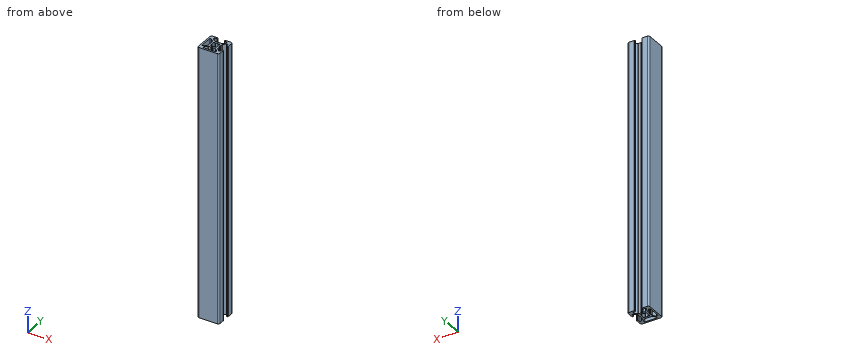
```python
from build123d import *

# Parameters (mm, degrees)
EXTRUDE1_DEPTH = 250


with BuildPart() as part:
    # Sketch1 → Extrude1 (new body)
    with BuildSketch(Plane.XY):
        with BuildLine():
            Line((-8.5, -10), (8.5, -10))
            ThreePointArc((8.5, -10), (9.560660172, -9.560660172), (10, -8.5))
            Line((10, -8.5), (10, -3.7))
            ThreePointArc((10, -3.7), (9.941421356, -3.558578644), (9.8, -3.5))
            Line((9.8, -3.5), (9.7, -3.5))
            ThreePointArc((9.7, -3.5), (9.558578644, -3.441421356), (9.5, -3.3))
            Line((9.5, -3.3), (9.5, -3.2))
            ThreePointArc((9.5, -3.2), (9.441421356, -3.058578644), (9.3, -3))
            Line((9.3, -3), (9, -3))
            ThreePointArc((9, -3), (8.646446609, -3.146446609), (8.5, -3.5))
            Line((8.5, -3.5), (8.5, -5.500000208))
            ThreePointArc((8.5, -5.500000208), (8.353553391, -5.853553598), (8, -6.000000208))
            Line((8, -6.000000208), (7.267767022, -6.000000208))
            ThreePointArc((7.267767022, -6.000000208), (7.076425294, -5.961939969), (6.914213614, -5.853553581))
            Line((6.914213614, -5.853553581), (4.646446828, -3.585786575))
            ThreePointArc((4.646446828, -3.585786575), (4.538060465, -3.423574906), (4.500000236, -3.232233201))
            Line((4.500000236, -3.232233201), (4.500000236, -0.953589838))
            ThreePointArc((4.500000236, -0.953589838), (4.493185401, -0.901826029), (4.473205317, -0.853589838))
            Line((4.473205317, -0.853589838), (4.038120021, -0.1))
            ThreePointArc((4.038120021, -0.1), (4.011325101, 0), (4.038120021, 0.1))
            Line((4.038120021, 0.1), (4.473205317, 0.853589838))
            ThreePointArc((4.473205317, 0.853589838), (4.493185401, 0.901826029), (4.500000236, 0.953589838))
            Line((4.500000236, 0.953589838), (4.500000236, 3.232233262))
            ThreePointArc((4.500000236, 3.232233262), (4.538060467, 3.423574973), (4.646446837, 3.585786644))
            Line((4.646446837, 3.585786644), (6.914213678, 5.853553596))
            ThreePointArc((6.914213678, 5.853553596), (7.076425355, 5.961939978), (7.267767077, 6.000000214))
            Line((7.267767077, 6.000000214), (8.000000112, 6.000000214))
            ThreePointArc((8.000000112, 6.000000214), (8.353553502, 5.853553604), (8.500000112, 5.500000214))
            Line((8.500000112, 5.500000214), (8.500000112, 3.5))
            ThreePointArc((8.500000112, 3.5), (8.646446721, 3.146446609), (9.000000112, 3))
            Line((9.000000112, 3), (9.300000112, 3))
            ThreePointArc((9.300000112, 3), (9.441421468, 3.058578644), (9.500000112, 3.2))
            Line((9.500000112, 3.2), (9.500000112, 3.3))
            ThreePointArc((9.500000112, 3.3), (9.558578756, 3.441421356), (9.700000112, 3.5))
            Line((9.700000112, 3.5), (9.8, 3.5))
            ThreePointArc((9.8, 3.5), (9.941421356, 3.558578644), (10, 3.7))
            Line((10, 3.7), (10, 8.5))
            ThreePointArc((10, 8.5), (9.560660172, 9.560660172), (8.5, 10))
            Line((8.5, 10), (3.7, 10))
            ThreePointArc((3.7, 10), (3.558578644, 9.941421356), (3.5, 9.8))
            Line((3.5, 9.8), (3.5, 9.7))
            ThreePointArc((3.5, 9.7), (3.441421356, 9.558578644), (3.3, 9.5))
            Line((3.3, 9.5), (3.2, 9.5))
            ThreePointArc((3.2, 9.5), (3.058578644, 9.441421356), (3, 9.3))
            Line((3, 9.3), (3, 9.000000069))
            ThreePointArc((3, 9.000000069), (3.146446609, 8.646446678), (3.5, 8.500000069))
            Line((3.5, 8.500000069), (5.550000287, 8.500000069))
            ThreePointArc((5.550000287, 8.500000069), (5.903553677, 8.353553459), (6.050000287, 8.000000069))
            Line((6.050000287, 8.000000069), (6.050000287, 7.267766898))
            ThreePointArc((6.050000287, 7.267766898), (6.011940051, 7.076425176), (5.903553669, 6.914213499))
            Line((5.903553669, 6.914213499), (3.635786717, 4.646446658))
            ThreePointArc((3.635786717, 4.646446658), (3.473575046, 4.538060288), (3.282233335, 4.500000057))
            Line((3.282233335, 4.500000057), (1.003589985, 4.500000057))
            ThreePointArc((1.003589985, 4.500000057), (0.951826176, 4.493185222), (0.903589985, 4.473205138))
            Line((0.903589985, 4.473205138), (0.150000146, 4.038119841))
            ThreePointArc((0.150000146, 4.038119841), (0.050000146, 4.011324922), (-0.049999854, 4.038119841))
            Line((-0.049999854, 4.038119841), (-0.803589692, 4.473205138))
            ThreePointArc((-0.803589692, 4.473205138), (-0.851825883, 4.493185222), (-0.903589692, 4.500000057))
            Line((-0.903589692, 4.500000057), (-3.182233104, 4.500000057))
            ThreePointArc((-3.182233104, 4.500000057), (-3.37357482, 4.538060291), (-3.535786494, 4.646446666))
            Line((-3.535786494, 4.646446666), (-5.803553391, 6.914213562))
            ThreePointArc((-5.803553391, 6.914213562), (-5.911939766, 7.076425237), (-5.95, 7.267766953))
            Line((-5.95, 7.267766953), (-5.95, 8))
            ThreePointArc((-5.95, 8), (-5.803553391, 8.353553391), (-5.45, 8.5))
            Line((-5.45, 8.5), (-3.5, 8.5))
            ThreePointArc((-3.5, 8.5), (-3.146446609, 8.646446609), (-3, 9))
            Line((-3, 9), (-3, 9.3))
            ThreePointArc((-3, 9.3), (-3.058578644, 9.441421356), (-3.2, 9.5))
            Line((-3.2, 9.5), (-3.35, 9.5))
            ThreePointArc((-3.35, 9.5), (-3.491421356, 9.558578644), (-3.55, 9.7))
            Line((-3.55, 9.7), (-3.55, 9.8))
            ThreePointArc((-3.55, 9.8), (-3.608578644, 9.941421356), (-3.75, 10))
            Line((-3.75, 10), (-8.5, 10))
            ThreePointArc((-8.5, 10), (-9.560660172, 9.560660172), (-10, 8.5))
            Line((-10, 8.5), (-10, -8.5))
            ThreePointArc((-10, -8.5), (-9.560660172, -9.560660172), (-8.5, -10))
        make_face()
        with BuildLine():
            Line((-5.500000147, -8.500000123), (5.500000242, -8.500000123))
            ThreePointArc((5.500000242, -8.500000123), (5.853553633, -8.353553514), (6.000000242, -8.000000123))
            Line((6.000000242, -8.000000123), (6.000000242, -7.267766878))
            ThreePointArc((6.000000242, -7.267766878), (5.961940006, -7.076425156), (5.853553624, -6.914213479))
            Line((5.853553624, -6.914213479), (3.585786637, -4.646446602))
            ThreePointArc((3.585786637, -4.646446602), (3.423574966, -4.538060233), (3.232233255, -4.500000001))
            Line((3.232233255, -4.500000001), (0.953589836, -4.500000001))
            ThreePointArc((0.953589836, -4.500000001), (0.901826025, -4.493185166), (0.853589832, -4.47320508))
            Line((0.853589832, -4.47320508), (0.100000004, -4.038119765))
            ThreePointArc((0.100000004, -4.038119765), (5e-09, -4.011324843), (-0.099999996, -4.03811976))
            Line((-0.099999996, -4.03811976), (-0.853589845, -4.473205038))
            ThreePointArc((-0.853589845, -4.473205038), (-0.901826034, -4.493185121), (-0.953589841, -4.499999955))
            Line((-0.953589841, -4.499999955), (-3.232233196, -4.499999955))
            ThreePointArc((-3.232233196, -4.499999955), (-3.423574907, -4.538060186), (-3.585786578, -4.646446556))
            Line((-3.585786578, -4.646446556), (-5.853553529, -6.914213397))
            ThreePointArc((-5.853553529, -6.914213397), (-5.961939911, -7.076425074), (-6.000000147, -7.267766796))
            Line((-6.000000147, -7.267766796), (-6.000000147, -8.000000123))
            ThreePointArc((-6.000000147, -8.000000123), (-5.853553538, -8.353553514), (-5.500000147, -8.500000123))
        make_face(mode=Mode.SUBTRACT)
        with BuildLine():
            Line((1.258185317, -2.445295423), (1.913894874, -2.989641056))
            ThreePointArc((1.913894874, -2.989641056), (2.510074363, -2.510074485), (2.989640962, -1.91389502))
            Line((2.989640962, -1.91389502), (2.445295362, -1.258185436))
            ThreePointArc((2.445295362, -1.258185436), (2.75, -6.7e-08), (2.445295423, 1.258185317))
            Line((2.445295423, 1.258185317), (2.989641056, 1.913894874))
            ThreePointArc((2.989641056, 1.913894874), (2.510074485, 2.510074363), (1.91389502, 2.989640962))
            Line((1.91389502, 2.989640962), (1.258185436, 2.445295362))
            ThreePointArc((1.258185436, 2.445295362), (6.7e-08, 2.75), (-1.258185317, 2.445295423))
            Line((-1.258185317, 2.445295423), (-1.913894874, 2.989641056))
            ThreePointArc((-1.913894874, 2.989641056), (-2.510074363, 2.510074485), (-2.989640962, 1.91389502))
            Line((-2.989640962, 1.91389502), (-2.445295362, 1.258185436))
            ThreePointArc((-2.445295362, 1.258185436), (-2.75, 6.7e-08), (-2.445295423, -1.258185317))
            Line((-2.445295423, -1.258185317), (-2.992174953, -1.909930962))
            ThreePointArc((-2.992174953, -1.909930962), (-2.511737261, -2.508410485), (-1.91389502, -2.989640962))
            Line((-1.91389502, -2.989640962), (-1.258185436, -2.445295362))
            ThreePointArc((-1.258185436, -2.445295362), (-6.7e-08, -2.75), (1.258185317, -2.445295423))
        make_face(mode=Mode.SUBTRACT)
        with BuildLine():
            Line((-8.5, -5.5), (-8.5, 5.50000039))
            ThreePointArc((-8.5, 5.50000039), (-8.353553351, 5.853553875), (-7.999999866, 6.000000524))
            Line((-7.999999866, 6.000000524), (-7.267766819, 6.000000524))
            ThreePointArc((-7.267766819, 6.000000524), (-7.076425092, 5.961940285), (-6.914213411, 5.853553897))
            Line((-6.914213411, 5.853553897), (-4.646446626, 3.585786891))
            ThreePointArc((-4.646446626, 3.585786891), (-4.538060262, 3.423575222), (-4.500000033, 3.232233517))
            Line((-4.500000033, 3.232233517), (-4.500000033, 0.953590154))
            ThreePointArc((-4.500000033, 0.953590154), (-4.493185199, 0.901826345), (-4.473205114, 0.853590154))
            Line((-4.473205114, 0.853590154), (-4.038119781, 0.100000251))
            ThreePointArc((-4.038119781, 0.100000251), (-4.011324861, 2.51e-07), (-4.038119781, -0.099999749))
            Line((-4.038119781, -0.099999749), (-4.473205138, -0.853589692))
            ThreePointArc((-4.473205138, -0.853589692), (-4.493185222, -0.901825883), (-4.500000057, -0.953589692))
            Line((-4.500000057, -0.953589692), (-4.500000057, -3.232233104))
            ThreePointArc((-4.500000057, -3.232233104), (-4.538060291, -3.42357482), (-4.646446666, -3.585786494))
            Line((-4.646446666, -3.585786494), (-6.914213562, -5.853553391))
            ThreePointArc((-6.914213562, -5.853553391), (-7.076425237, -5.961939766), (-7.267766953, -6))
            Line((-7.267766953, -6), (-8, -6))
            ThreePointArc((-8, -6), (-8.353553391, -5.853553391), (-8.5, -5.5))
        make_face(mode=Mode.SUBTRACT)
    extrude(amount=EXTRUDE1_DEPTH)


solid = part.part
```
Build history of the part. All positions in model axes, mm. Give positions to 0.01 mm unless a question says otherwise; leave off trailing zeros. One line per question, with ' | ' between items.
Q1. Cut at A-A, the plane z = 40.5. Count the separate pieces of the cut face and the enclosed holes in it, plus the area to 3 significant figures.
Filled sheet:
separate pieces: 1 | enclosed holes: 3 | area: 183 mm²
Q2. Drop flat-ended pins along their axis: pin 1 (3.5 mm diameter, centred on x = -2, z = 181, fed in from +Y); pin 2 (5.5 mm diameter, centred on y = 0, z = 125, fed in from +X); pin 3 (1.5 mm diameter, centred on x = 7.5, y = -1.5, fed in from -Z). Give the stop position or say it passes through.
Filled sheet:
pin 1: stops at y = 10 | pin 2: stops at x = 4.5 | pin 3: passes through
Q3. Drill centre lines: line 1 along X through (y, z) = (4.25, 115); line 2 along Y through (x, z) = (7.75, 47.5); line 3 along X through (y, z) = (2, 17). Where is each one in solid material? Low to high. Write a range as [from, to].
Filled sheet:
line 1: x = [-10, -8.5], [-5.31, -0.42], [0.52, 5.31], [8.5, 10] | line 2: y = [-10, -6], [6, 10] | line 3: x = [-10, -8.5], [-4.5, -2.93], [2.93, 4.5]
